Can you work these out from the model? Positions are in its coordinate system, mm. A direction names the side the tool comes from. Round coordinates to 2 decimals unless told otherwise and drop trailing zeros. Loops run counter-clockwise (first coordinate to the right, second up) from the corner with the lowest first, then second, coordinate; pieces in that order, holes last. Notation, with made-up numbers: (47.5, 42) -> (103.5, 42) arc R15 ccw to (103.5, 71) -> close; hole circle Ø9 at (32, -33). An arc over 180 degrees is marked (long way). Write each question's results on one line, items separated by ' | '.
from build123d import *

# Parameters (mm, degrees)
F0_R     = 76.2
F0_R_2   = 3.175
F1_DEPTH = 19.05
F3_DEPTH = 6.35


with BuildPart() as f1:
    # F0 (on Top) → F1 (new body)
    with BuildSketch(Plane.XY):
        Circle(F0_R)
        Circle(F0_R_2, mode=Mode.SUBTRACT)
    extrude(amount=F1_DEPTH)

    # F2 (on face) → F3 (cut)
    with BuildSketch(Plane.XY.offset(19.05)):
        Polygon((9.652, 38.927315), (-9.652, 38.927315), (-55.5625, -29.678286), (55.5625, -29.678286), align=None)
    extrude(amount=-F3_DEPTH, mode=Mode.SUBTRACT)


solid = f1.part
1. If we section it at C-C (z = 8.75): List the corners of the cut face in (x, y) for me (3 decimals), then the cut area to 3 significant figures.
Final values:
outline: circle Ø152.4 at (0, 0); hole circle Ø6.35 at (0, 0) | area: 18,200 mm2
2. If we section it at D-D (y = 35.5): List the corners of the cut face in (x, z) for me.
Final values:
outline: (-67.43, 0) -> (67.43, 0) -> (67.43, 19.05) -> (11.95, 19.05) -> (11.95, 12.7) -> (-11.95, 12.7) -> (-11.95, 19.05) -> (-67.43, 19.05) -> close
3. Will these pins go through, and if not, where does the flat tip stop? pin 1 (2 mm diameter, centred on x = 34.5, z = 6.5, fed in from +Y); pin 2 (1.5 mm diameter, centred on x = -42.5, z = 12, fed in from +Y); pin 3 (1.9 mm diameter, centred on x = -6.5, z = 14.5, fed in from +Y).
Final values:
pin 1: y = 68.44 | pin 2: y = 63.74 | pin 3: y = 76
4. On a 3-axis mill with a long thin cutter (end or side, diameter ignored), from which of +Z, -Z, +X, -X, +Y, -Y can I reach the whole of each face in a straight line? I mean faces 4 (the face through (-1, -33, 19.05)), 5 (the face through (-32.29, 5.1, 15.92)). Say none if no direction works.
Final values:
face 4: +Z, +X, -X, +Y, -Y | face 5: +Z
5. We'd pull the mould along Y, two halves only. Please class faces 1 (the face through (-60.47, -46.367, 9.392)), 2 (the face through (-1, -29.678, 16)), 3 (the face through (16, 1, 0)): pulls with the +Y half, pulls with the -Y half, needs draft (parallel to the pull), parting line crosses it, or undercut.
Final values:
face 1: parting line crosses it | face 2: undercut | face 3: needs draft
6. If we section it at B-B (y = 0): List the corners of the cut face in (x, z) for me (3 decimals).
Final values:
outline: (-76.2, 0) -> (-3.175, 0) -> (-3.175, 12.7) -> (-35.702, 12.7) -> (-35.702, 19.05) -> (-76.2, 19.05) -> close; (3.175, 0) -> (76.2, 0) -> (76.2, 19.05) -> (35.702, 19.05) -> (35.702, 12.7) -> (3.175, 12.7) -> close
7. If we section it at A-A (x = 0): List the corners of the cut face in (y, z) for me (3 decimals), then the cut area to 3 significant figures.
Final values:
outline: (-76.2, 0) -> (-3.175, 0) -> (-3.175, 12.7) -> (-29.678, 12.7) -> (-29.678, 19.05) -> (-76.2, 19.05) -> close; (3.175, 0) -> (76.2, 0) -> (76.2, 19.05) -> (38.927, 19.05) -> (38.927, 12.7) -> (3.175, 12.7) -> close | area: 2,390 mm2
8. Please list where these lines run through material, in increasing order: line 1 (Y direction, x = 0, z = 8) (3 decimals); line 2 (Z direction, x = -8, y = 32); line 3 (Y direction, x = -1, z = 3). Write a range as from..to.
Final values:
line 1: -76.2..-3.175, 3.175..76.2 | line 2: 0..12.7 | line 3: -76.19..-3.01, 3.01..76.19
